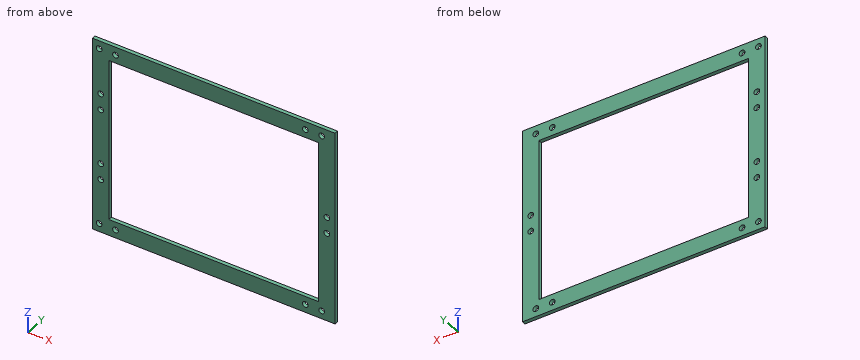
```python
from build123d import *

# Parameters (mm, degrees)
SKETCH1_W           = 296
SKETCH1_H           = 240
SKETCH1_W_2         = 256
SKETCH1_H_2         = 200
BOSS_EXTRUDE1_DEPTH = 4.5
SKETCH2_R           = 3.5
CUT_EXTRUDE1_DEPTH  = 4.5
SKETCH3_R           = 3.5
CUT_EXTRUDE2_DEPTH  = 4.5
SKETCH4_R           = 3.5
CUT_EXTRUDE3_DEPTH  = 4.5
SKETCH5_R           = 3.5
CUT_EXTRUDE4_DEPTH  = 4.5


with BuildPart() as part:
    # Sketch1 → Boss-Extrude1 (new body)
    with BuildSketch(Plane(origin=(0, 0, 0), x_dir=(1, 0, 0), z_dir=(0, 1, 0))):
        Rectangle(SKETCH1_W, SKETCH1_H)
        Rectangle(SKETCH1_W_2, SKETCH1_H_2, mode=Mode.SUBTRACT)
    extrude(amount=BOSS_EXTRUDE1_DEPTH)

    # Sketch2 → Cut-Extrude1 (cut)
    with BuildSketch(Plane(origin=(0, 4.5, 0), x_dir=(1, 0, 0), z_dir=(0, 1, 0))):
        with Locations((-139.9, -110)):
            Circle(SKETCH2_R)
        with Locations((-119.9, -110)):
            Circle(SKETCH2_R)
    cut_extrude1 = extrude(amount=-CUT_EXTRUDE1_DEPTH, mode=Mode.SUBTRACT)

    # Mirror1: Cut-Extrude1 across plane
    add(cut_extrude1.mirror(Plane.XY), mode=Mode.SUBTRACT)

    # Sketch3 → Cut-Extrude2 (cut)
    with BuildSketch(Plane(origin=(0, 4.5, 0), x_dir=(1, 0, 0), z_dir=(0, 1, 0))):
        with Locations((131.7, -110)):
            Circle(SKETCH3_R)
        with Locations((111.7, -110)):
            Circle(SKETCH3_R)
    cut_extrude2 = extrude(amount=-CUT_EXTRUDE2_DEPTH, mode=Mode.SUBTRACT)

    # Mirror2: Cut-Extrude2 across plane
    add(cut_extrude2.mirror(Plane.XY), mode=Mode.SUBTRACT)

    # Sketch4 → Cut-Extrude3 (cut)
    with BuildSketch(Plane(origin=(0, 4.5, 0), x_dir=(1, 0, 0), z_dir=(0, 1, 0))):
        with Locations((138, 10)):
            Circle(SKETCH4_R)
        with Locations((138, -10)):
            Circle(SKETCH4_R)
    extrude(amount=-CUT_EXTRUDE3_DEPTH, mode=Mode.SUBTRACT)

    # Sketch5 → Cut-Extrude4 (cut)
    with BuildSketch(Plane(origin=(0, 4.5, 0), x_dir=(1, 0, 0), z_dir=(0, 1, 0))):
        with Locations((-138, 53.924043482)):
            Circle(SKETCH5_R)
        with Locations((-138, 33.924043482)):
            Circle(SKETCH5_R)
        with Locations((-138, -33.924043482)):
            Circle(SKETCH5_R)
        with Locations((-138, -53.924043482)):
            Circle(SKETCH5_R)
    extrude(amount=-CUT_EXTRUDE4_DEPTH, mode=Mode.SUBTRACT)


solid = part.part
```
Geometry check sheet. Reference: the model listing, model coordinates, mm. Coordinates: 2 decimals unless noted, no trailing zeros. Order: outer loops, then holes, each group sorted by start corner. A loop starts at its lowest first (then second) coordinate and runs counter-clockwise, first axis right, second up. Notation, with made-up numbers: M -12,-18 L -4,-18 A22 cw -4,16 Z; hole C 16.5,21.5 d1. An arc over 180 degrees is marked long. One line per question, with ' | ' between items. Start each with the question number.
Item 1: Gauge pin test, flat ends, axial feed: pin 1 (6.5 mm diameter, centred on x = -138, z = 53.92, fed in from +Y); pin 2 (11 mm diameter, centred on x = -119.9, z = 110, fed in from +Y). Record the tip position at first contact, or that the pin passes through.
Item 2: Cross-section at B-B on x = -35. Enter the section's corners in (y, z), then the cut area to 3 significant figures.
Item 3: Material ranges on L1, parallel to Z at x = 131.7, y = 3.05; L2, parallel to Z at x = 138, y = 2.95; L3, parallel to Z at x = -119.9, y = 1.35, recorded low to high. Write a range as [from, to].
Item 4: Cross-section at C-C on z = 64. Enter the section's corners in (x, y), then the cut area to 3 significant figures.
Item 5: Cross-section at A-A on z = -110. Enter the section's corners in (x, y).
Item 6: Cross-section at D-D on z = -10. Enter the section's corners in (x, y).
Findings:
1) pin 1: passes through | pin 2: stops at y = 4.5
2) outline: M 0,-120 L 4.5,-120 L 4.5,-100 L 0,-100 Z; M 0,100 L 4.5,100 L 4.5,120 L 0,120 Z | area: 180 mm²
3) L1: z = [-120, -113.5], [-106.5, 106.5], [113.5, 120] | L2: z = [-120, -13.5], [-6.5, 6.5], [13.5, 120] | L3: z = [-120, -113.5], [-106.5, -100], [100, 106.5], [113.5, 120]
4) outline: M -148,0 L -128,0 L -128,4.5 L -148,4.5 Z; M 128,0 L 148,0 L 148,4.5 L 128,4.5 Z | area: 180 mm²
5) outline: M -148,0 L -143.4,0 L -143.4,4.5 L -148,4.5 Z; M -136.4,0 L -123.4,0 L -123.4,4.5 L -136.4,4.5 Z; M -116.4,0 L 108.2,0 L 108.2,4.5 L -116.4,4.5 Z; M 115.2,0 L 128.2,0 L 128.2,4.5 L 115.2,4.5 Z; M 135.2,0 L 148,0 L 148,4.5 L 135.2,4.5 Z
6) outline: M -148,0 L -128,0 L -128,4.5 L -148,4.5 Z; M 128,0 L 134.5,0 L 134.5,4.5 L 128,4.5 Z; M 141.5,0 L 148,0 L 148,4.5 L 141.5,4.5 Z
